```python
from build123d import *

# Parameters (mm, degrees)
BOSS_EXTRUDE1_DEPTH = 1
BOSS_EXTRUDE2_START = -1
BOSS_EXTRUDE2_DEPTH = 5


with BuildPart() as part:
    # Sketch1 → Boss-Extrude1 (new body)
    with BuildSketch(Plane.XY):
        with BuildLine():
            Line((33.25, 27), (-33.25, 27))
            Line((-33.25, 27), (-33.25, -27))
            Line((-33.25, -27), (33.25, -27))
            Line((33.25, -27), (33.25, -10.816653826))
            ThreePointArc((33.25, -10.816653826), (-5.75, 0), (33.25, 10.816653826))
            Line((33.25, 10.816653826), (33.25, 27))
        make_face()
    extrude(amount=BOSS_EXTRUDE1_DEPTH)

    # Sketch2 → Boss-Extrude2 (add)
    with BuildSketch(Plane.XY.offset(1).offset(BOSS_EXTRUDE2_START)):
        Polygon((33.25, -19), (32.25, -19), (32.25, -26), (-32.25, -26), (-32.25, -19), (-33.25, -19), (-33.25, -27), (33.25, -27), align=None)
        Polygon((33.25, 27), (-33.25, 27), (-33.25, 19), (-32.25, 19), (-32.25, 26), (32.25, 26), (32.25, 19), (33.25, 19), align=None)
    extrude(amount=-BOSS_EXTRUDE2_DEPTH)


solid = part.part
```
Geometry: final body of the model. Coordinates: model frame, mm. A direction names the side the tool comes from. Round coordinates to 2 decimals unless told otherwise and drop trailing zeros. Write each loop counter-clockwise with the first axis right and the second up, starting at its lowest first coordinate (ties: lowest second). Pieces come first, ordered by that corner, then holes. Notation, with made-up numbers: (-28.5, 84.25) -> (-4.5, 84.25) arc R16 cw to (-4.5, 95.25) -> close; hole circle Ø11 at (-30.5, 65.5). An arc over 180 degrees is marked (long way). Use CSV: the item, a comma, the result in double quotes. Start each with the question number.
Q1. Section B-B (z = -1.55). Return loops of the section in (x, y).
Q2. Section A-A (x = 15.25). Return loops of the section in (y, z), plus the area to 3 significant figures.
Q3. First-contact query: pin 1 Ø1.5 at (x, y) = (-25, -14.5) entering from -Z. Flat tip, straight axial feed; report the tip coordinate or a pass-through.
Q4. Reachability of faces 1 (the face through (-33.25, 0.1, 0.2)), 2 (the face through (-32.25, 22, -2)) from +Z, -Z, +X, -X, +Y, -Y: full face, straight path, thin tool, end or side. Return the list, or none.
Q5. Section C-C (y = -23). Return loops of the section in (x, z).
Q6. Section D-D (x = 27.5). Return loops of the section in (y, z), plus the area to 3 significant figures.
Q7. Line query: L1, parallel to Y at x = 4, z = -0.35; L2, parallel to Y at x = 15.25, z = 0.2; L3, parallel to X at y = 24, z = -0.8. Output: solid intervals per line, ascending.
Result sheet:
1,outline,"(-33.25, -27) -> (33.25, -27) -> (33.25, -19) -> (32.25, -19) -> (32.25, -26) -> (-32.25, -26) -> (-32.25, -19) -> (-33.25, -19) -> close; (-33.25, 19) -> (-32.25, 19) -> (-32.25, 26) -> (32.25, 26) -> (32.25, 19) -> (33.25, 19) -> (33.25, 27) -> (-33.25, 27) -> close"
2,outline,"(-27, -5) -> (-26, -5) -> (-26, 0) -> (-21, 0) -> (-21, 1) -> (-27, 1) -> close; (21, 0) -> (26, 0) -> (26, -5) -> (27, -5) -> (27, 1) -> (21, 1) -> close"
2,area,"22.0 mm²"
3,pin 1,"z = 0"
4,face 1,"+Z, -Z, -X, +Y, -Y"
4,face 2,"-Z"
5,outline,"(-33.25, -5) -> (-32.25, -5) -> (-32.25, 0) -> (32.25, 0) -> (32.25, -5) -> (33.25, -5) -> (33.25, 1) -> (-33.25, 1) -> close"
6,outline,"(-27, -5) -> (-26, -5) -> (-26, 0) -> (-17.06, 0) -> (-17.06, 1) -> (-27, 1) -> close; (17.06, 0) -> (26, 0) -> (26, -5) -> (27, -5) -> (27, 1) -> (17.06, 1) -> close"
6,area,"29.9 mm²"
7,L1,"-27 to -26, 26 to 27"
7,L2,"-27 to -21, 21 to 27"
7,L3,"-33.25 to -32.25, 32.25 to 33.25"
